from build123d import *

# Parameters (mm, degrees)
F0_W     = 81.5
F0_H     = 150
F1_DEPTH = 40.5
F2_R     = 2.38125
F3_DEPTH = 10


with BuildPart() as f1:
    # F0 (on Top) → F1 (new body)
    with BuildSketch(Plane.XY):
        Rectangle(F0_W, F0_H)
    extrude(amount=F1_DEPTH)

    # F2 (on face) → F3 (cut)
    with BuildSketch(Plane.XZ.offset(75)):
        with Locations((35.15, 36.1)):
            Circle(F2_R)
        with Locations((35.15, 4.1)):
            Circle(F2_R)
        with Locations((3.15, 36.1)):
            Circle(F2_R)
    extrude(amount=-F3_DEPTH, mode=Mode.SUBTRACT)


solid = f1.part
Input: part model. Units: mm. Frame: model coordinates. A direction names the side the tool comes from. Coordinates: 2 decimals unless noted, no trailing zeros. Loops run counter-clockwise (first coordinate to the right, second up) from the corner with the lowest first, then second, coordinate; pieces in that order, holes last.
Q1. Contact query for flat-ended pins moving along their axis: pin 1 (1.4 mm diameter, centred on x = 36, z = 36.5, fed in from -Y); pin 2 (12 mm diameter, centred on x = 11, y = 47, fed in from -Z). Output: stop coordinate, or through.
Q2. Material intervals for line 1 (X direction, y = -70, z = 36); line 2 (Z direction, x = 35, y = -70); line 3 (Z direction, x = 3.15, y = -68.75), sorted ascending.
Q3. Set-up query: faces 4 (the face through (35, -65, 36)), 5 (the face through (-1, 75, 20)). Return all of +Z, -Z, +X, -X, +Y, -Y with unobstructed straight access to the full face (end or side cutting, diameter ignored); none if empty.
Q4. Draft query along X for faces 1 (the face through (-40.75, -1, 20)), 2 (the face through (-1, -75, 20)), 3 (the face through (35, -65, 4)). Return one class per face: +X half, -X half, draft (parallel to the pull), parting line (faces both ways), or undercut.
Q5. Cut plane A-A (x = 35.15). Output: boundary loops of the cut face in (y, z).
Working result:
1. pin 1: stops at y = -65
1. pin 2: stops at z = 0
2. line 1: x = -40.75 to 0.77, 5.53 to 32.77, 37.53 to 40.75
2. line 2: z = 0 to 1.72, 6.48 to 33.72, 38.48 to 40.5
2. line 3: z = 0 to 33.72, 38.48 to 40.5
3. face 4: -Y
3. face 5: +Z, -Z, +X, -X, +Y
4. face 1: -X half
4. face 2: draft
4. face 3: undercut
5. outline: (-75, 0) - (75, 0) - (75, 40.5) - (-75, 40.5) - (-75, 38.48) - (-65, 38.48) - (-65, 33.72) - (-75, 33.72) - (-75, 6.48) - (-65, 6.48) - (-65, 1.72) - (-75, 1.72) - close
